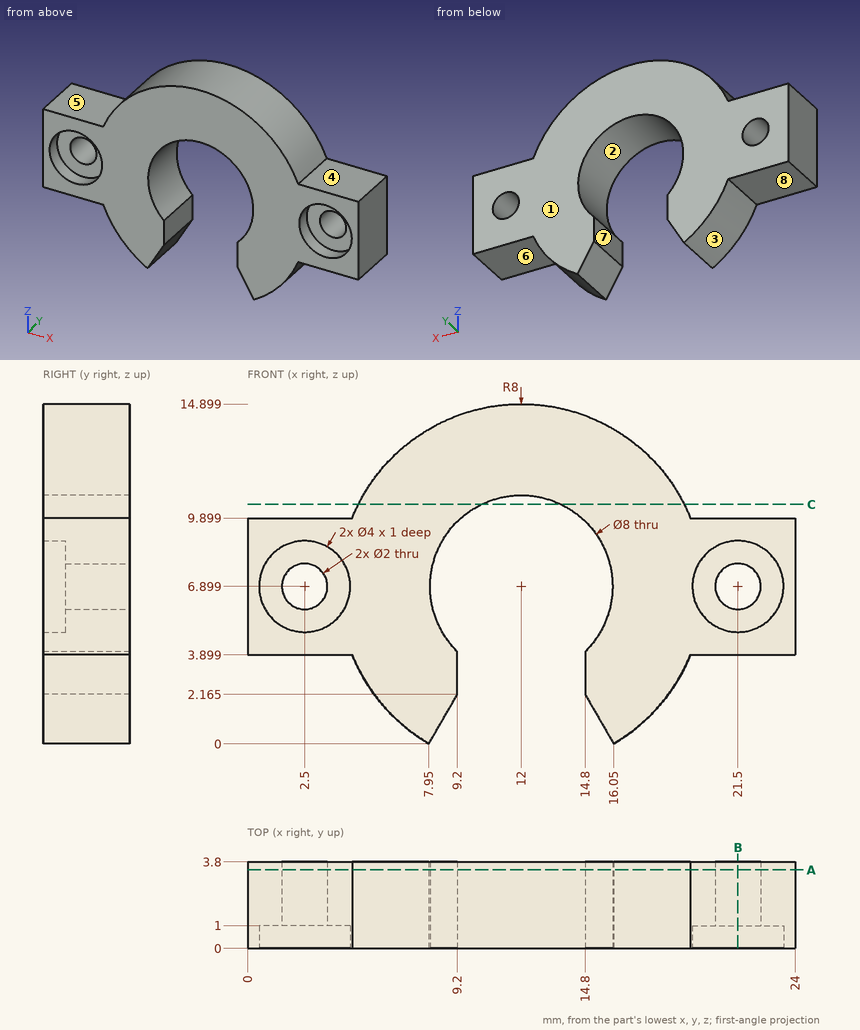
The figure shows three views and two pictorial views of one solid part (mm, origin at its lowest corner). Answer the questions. A direction names the side the tool comes from. Round coordinates to 2 decimals unless told otherwise and drop trailing zeros. Loops run counter-clockwise (first coordinate to the right, second up) from the corner with the lowest first, then second, coordinate; pieces in that order, holes last. Notation, with made-up numbers: (60.25, 6) -> (97.25, 6) arc R15 ccw to (97.25, 14) -> close; hole circle Ø3 at (26.25, 80). An arc over 180 degrees is marked (long way). Use one line per item in the form item = value.
(1) Find section A-A on y = 3.45. Give the number of separate pieces and of enclosed holes in the cut face, then the cut area to 3 significant figures.
Answer list:
separate_pieces = 1
enclosed_holes = 2
area = 168 mm2
(2) A tool of negligible diameter and unlimited length cuts with its end or side. For the marked faces 4, 5, 6, 7 and 8, from which of +Z, -Z, +X, -X, +Y, -Y can it reach the whole face along a straight path? Write none if from no direction.
Answer list:
face_4 = +Z, +X, +Y, -Y
face_5 = +Z, -X, +Y, -Y
face_6 = -Z, +X, +Y, -Y
face_7 = -Z, +Y, -Y
face_8 = -Z, -X, +Y, -Y
(3) For a pull along X with two mould halves and no side action, classify the marked faces 1, 2 and 3 as released by +X, released by -X, zero draft, split by the parting line, or undercut.
Answer list:
face_1 = zero draft
face_2 = undercut
face_3 = released by -X
(4) Find section C-C on z = 10.5. Give the vertices of the cut face in (x, y).
Answer list:
outline = (4.86, 0) -> (10.26, 0) -> (10.26, 3.8) -> (4.86, 3.8) -> close; (13.74, 0) -> (19.14, 0) -> (19.14, 3.8) -> (13.74, 3.8) -> close
(5) Straight lines are drawn through the part: line 1 (X direction, y = 2.65, z = 7) (1 decimal); line 2 (X direction, y = 0.35, z = 7.25); line 3 (Z direction, x = 21.5, y = 1.7). For each, find the intervals that lie inside material, in ascending order.
Answer list:
line_1 = 0 to 1.5, 3.5 to 8, 16 to 20.5, 22.5 to 24
line_2 = 0 to 0.53, 4.47 to 8.02, 15.98 to 19.53, 23.47 to 24
line_3 = 3.9 to 5.9, 7.9 to 9.9
(6) Flat-ended cylindrical pins translate along their axes: P1, Ø1.1, axis at x = 1.5, y = 1.5, coming from the +Z side; P2, Ø1.9, axis at x = 21, y = 1.5, coming from the -Z side; P3, Ø2.5, axis at x = 2.5, z = 6.9, coming from the -Y side. Find the tip coordinate at first contact, or state that the pin passes through.
Answer list:
P1 = 9.9
P2 = 3.9
P3 = 1
(7) Find section B-B on x = 21.5. Give the vertices of the cut face in (y, z).
Answer list:
outline = (0, 3.9) -> (3.8, 3.9) -> (3.8, 5.9) -> (1, 5.9) -> (1, 4.9) -> (0, 4.9) -> close; (0, 8.9) -> (1, 8.9) -> (1, 7.9) -> (3.8, 7.9) -> (3.8, 9.9) -> (0, 9.9) -> close
